Autodesk Inventor part; units mm, degrees
ref_plane "YZ Plane" through (0, 0, 0) normal (1, 0, 0) x (0, 1, 0)
ref_plane "XZ Plane" through (0, 0, 0) normal (0, 1, 0) x (-1, 0, 0)
ref_plane "XY Plane" through (0, 0, 0) normal (0, 0, 1) x (1, 0, 0)
sketch "Sketch1 outline for Plate1" plane through (0, 0, 0) normal (0, 0, 1) x (1, 0, 0)
  line L0 (0, 106.3625) -> (0, 0)
  line L1 (41.275, 106.3625) -> (0, 106.3625)
  line L2 (0, 0) -> (41.275, 0)
  line L3 (41.275, 0) -> (41.275, 106.3625)
  circle A0 centre (9.525, 12.7) radius 2.0701
  circle A1 centre (12.7, 38.1) radius 2.0701
  circle A2 centre (34.925, 12.7) radius 2.0701
  circle A3 centre (12.7, 63.5) radius 2.0701
  circle A4 centre (12.7, 88.9) radius 2.0701
extrude "Plate1" add sketch "Sketch1 outline for Plate1" along normal blind 3.175
sketch "Sketch2" plane through (0, 107.6325, 4.445) normal (0, 1, 0) x (-1, 0, 0)
  line L0 (-41.275, 0) -> (0, 0)
  line L1 (0, 0) -> (0, 20.955)
  line L2 (0, 20.955) -> (-41.275, 20.955)
  line L3 (-41.275, 20.955) -> (-41.275, 0)
edge flange "Flange1" height 25.4 angle 90 thickness 3.175 bend radius 1.27 thickness toward (0, 1, 0) relief tear relief width 3.175 relief depth 1.5875 edges at (20.6375, 106.3625, 3.175) wall of the first edge with corners at (41.275, 107.6325, 4.445) (0, 107.6325, 4.445) (0, 107.6325, 25.4) (41.275, 107.6325, 25.4)
bend "Bend1"
corner "Corner1"
sketch "Sketch1" plane through (0, 0, 0) normal (0, 0, 1) x (1, 0, 0)
  line L0 (110.551814, -41.275) -> (0, -41.275)
  line L1 (110.551814, -34.925) -> (110.551814, -41.275)
  line L2 (0, 0) -> (111.304505, 0)
  line L3 (106.3625, 0) -> (110.551814, 0)
  line L4 (110.551814, 0) -> (110.551814, -3.175)
  line L5 (110.551814, -3.175) -> (106.3625, -3.175)
  line L6 (106.3625, -3.175) -> (106.3625, 0)
  line L7 (106.3625, 0) -> (106.3625, -41.275)
  line L8 (110.551814, 0) -> (110.551814, -34.925)
  line L9 (106.3625, -38.1) -> (110.551814, -38.1)
  line L10 (110.551814, -38.1) -> (110.551814, -41.275)
  line L11 (110.551814, -41.275) -> (106.3625, -41.275)
  line L12 (106.3625, -41.275) -> (106.3625, -38.1)
  dimension "d6" = 25.4
  dimension "d22" = 12.7
  dimension "d36" = 6.35
  dimension "d38" = 12.7
  dimension "d39" = 38.1
  dimension "d42" = 25.4
sketch "Sketch4" plane through (0, 110.8075, 25.4) normal (0, 1, 0) x (1, 0, 0)
  line L0 (41.275, 0) -> (0, 0)
  circle A0 centre (19.05, 6.35) radius 2.3749
  line L1 (0, 0) -> (0, 20.955)
  line L2 (0, 20.955) -> (41.275, 20.955)
  line L3 (41.275, 20.955) -> (41.275, 21.413463)
  line L4 (21.135301, 0) -> (22.225, 0)
  line L5 (0, 0) -> (0, 20.955)
  line L6 (41.275, 20.955) -> (0, 20.955)
  line L7 (41.275, 20.955) -> (41.275, 17.78)
  line L8 (41.275, 17.78) -> (28.240357, 3.1812)
  line L9 (12.7, 9.525) -> (12.7, 20.955)
  arc A1 (12.7, 9.525) -> (21.68015, 0.015596) centre (22.225, 9.525) ccw
  arc A2 (21.68015, 0.015596) -> (28.240357, 3.1812) centre (21.135301, 9.525) ccw
  line L10 (41.275, 20.955) -> (41.275, 0)
  line L11 (0, 0) -> (41.275, 0)
  line L12 (41.275, 0) -> (41.275, 20.955)
  point P0 (0, 25.4)
  point P1 (12.7, 0)
  point P2 (25.4, 0)
  point P3 (12.7, 0)
  dimension "d28" = 4.7498
  dimension "d29" = 6.35
  dimension "d34" = 19.05
  dimension "d47" = 3.175
  dimension "d48" = 6.35
  dimension "d49" = 6.35
  dimension "d50" = 9.525
extrude "Cut3" cut sketch "Sketch4" against normal blind 3.175 contours L0 L1 L2 L9 A1 A2 L8 L10 | A0
fillet "Fillet3" radius 6.35 2 edges at (41.275, 109.22, 7.62) (12.7, 109.22, 4.445)
equation "\"d51\" = Thickness"
equation "\"d12\" = BendReliefWidth"
equation "\"d13\" = BendReliefDepth"
equation "\"d14\" = MinimumRemnant"
equation "\"d15\" = BendRadius"
equation "\"d19\" = CornerReliefSize"
equation "\"d20\" = GapSize"
equation "\"d21\" = JacobiRadiusSize"
equation "\"BendRadius\" = Thickness"
equation "\"BendReliefWidth\" = Thickness"
equation "\"BendReliefDepth\" = 0.5 * Thickness"
equation "\"CornerReliefSize\" = 4 * Thickness"
equation "\"MinimumRemnant\" = 2 * Thickness"
equation "\"TransitionRadius\" = BendRadius"
equation "\"JacobiRadiusSize\" = BendRadius"
equation "\"GapSize\" = Thickness"
equation "\"d11\" = BendRadius"
properties part number "Pneumatic Piston Front Flange (Left Custom)" material "Aluminum 6061"
Model file for the job. Use its own axes, mm. A direction names the side the tool comes from. Coordinates: 2 decimals unless noted, no trailing zeros. Order: outer loops, then holes, each group sorted by start corner. A loop starts at its lowest first (then second) coordinate and runs counter-clockwise, first axis right, second up. Notation, with made-up numbers: (-5.5, 4) -> (10.5, 4) arc R19 ccw to (10.5, 36) -> close; hole circle Ø10 at (-10.75, 9.25). An arc over 180 degrees is marked (long way). Answer as a JSON object with one key per item and string values. Group by question number.
1) Cut at A-A, the plane y = 38.1. Write the cut outline in (x, z) (3 decimals), then the cut area to 3 significant figures.
2) Flat gauge pins, fed straight in: pin 1 (2.5 mm diameter, centred on x = 2, y = 109, fed in from +Z) (3 decimals); pin 2 (1.5 mm diameter, centred on x = 17.5, z = 3, fed in from +Y); pin 3 (1 mm diameter, centred on x = 17, z = 13.5, fed in from -Y); pin 4 (2.5 mm diameter, centred on x = 9.525, y = 12.7, fed in from +Z). Where does each tip first touch, or does it go through?
3) Cut at D-D, the plane y = 25.5. Write the cut outline in (x, z) (3 decimals), then the cut area to 3 significant figures.
4) Pull direction X, two halves, no side cores. Call faces 1 (the face through (24, 107.632, 12)), 2 (the face through (20.146, 109.242, 21.157)), 3 (the face through (0, 56, 2)): +X half, -X half, draft (parallel to the pull), parting line (faces both ways), or undercut.
5) Cut at C-C, the plane x = 35.5. Write the cut outline in (y, z) (1 decimal), then the cut area to 3 significant figures.
6) Cut at B-B, the plane y = 12.7. Write the cut outline in (x, z) (3 decimals).
7) Drill centre lines: L1, parallel to Y at x = 12.7, z = 0.7; L2, parallel to Y at x = 12.7, z = 2.1; L3, parallel to Z at x = 25, y = 84 (3 decimals). Where is each one in solid material? Low to high.
8) Which spindle directions (+Z, -Z, +X, -X, +Y, -Y) get a long thin tool onto all of the face, cutting with end or side? Do faces 4 (the face through (12.7, 109, 13)), 5 (the face through (25.228, 109.242, 24.476)). Say none if no direction does.
Check values:
{
 "1": {"outline": "(0, 0) -> (10.63, 0) -> (10.63, 3.175) -> (0, 3.175) -> close; (14.77, 0) -> (41.275, 0) -> (41.275, 3.175) -> (14.77, 3.175) -> close", "area": "118 mm²"},
 "2": {"pin 1": "stops at z = 4.445", "pin 2": "stops at y = 110.75", "pin 3": "stops at y = 107.63", "pin 4": "passes through"},
 "3": {"outline": "(0, 0) -> (41.275, 0) -> (41.275, 3.175) -> (0, 3.175) -> close", "area": "131 mm²"},
 "4": {"face 1": "draft", "face 2": "undercut", "face 3": "-X half"},
 "5": {"outline": "(0, 0) -> (10.7, 0) -> (10.7, 3.2) -> (0, 3.2) -> close; (14.7, 0) -> (106.4, 0) arc R4.4 ccw to (110.8, 4.4) -> (110.8, 14.1) -> (107.6, 14.1) -> (107.6, 4.4) arc R1.3 cw to (106.4, 3.2) -> (14.7, 3.2) -> close", "area": "370 mm²"},
 "6": {"outline": "(0, 0) -> (7.455, 0) -> (7.455, 3.175) -> (0, 3.175) -> close; (11.595, 0) -> (32.855, 0) -> (32.855, 3.175) -> (11.595, 3.175) -> close; (36.995, 0) -> (41.275, 0) -> (41.275, 3.175) -> (36.995, 3.175) -> close"},
 "7": {"L1": "y = 0 to 36.03, 40.17 to 61.43, 65.57 to 86.83, 90.97 to 108.76", "L2": "y = 0 to 36.03, 40.17 to 61.43, 65.57 to 86.83, 90.97 to 110.14", "L3": "z = 0 to 3.175"},
 "8": {"face 4": "+Z, -X, +Y, -Y", "face 5": "+Z, +X, +Y, -Y"}
}
